Input: part model. Units: mm. Frame: model coordinates. A direction names the side the tool comes from. Coordinates: 2 decimals unless noted, no trailing zeros. Write each loop counter-clockwise with the first axis right and the second up, starting at its lowest first coordinate (ties: lowest second). Pieces come first, ordered by that corner, then holes. Notation, with made-up numbers: (19, -21) -> (42, -21) arc R16 ccw to (42, -13) -> close; hole circle Ø1 at (-6.5, -28.75). An arc over 180 degrees is marked (long way). Use one line per item in the form item = value. Start each with the question number.
(1) Cut plane B-B on y = 20.5. Return the cut outline in (x, z).
(2) Ray query, line 1 along X through (y, z) = (-43, 30); line 2 along X through (y, z) = (-16.5, 34.5); line 3 along X through (y, z) = (-49.5, 23.5). Return the intervals inside material, ascending.
(3) Cut plane A-A on x = -52.5. Return the cut outline in (y, z), plus the area to 3 significant figures.
(4) Cut plane D-D on y = 48.5. Return the cut outline in (x, z), plus the area to 3 significant figures.
(5) Set-up query: faces 5 (the face through (29.11, 26.443, 19.72)), 6 (the face through (63.35, -12.65, 20.28)). Return all of +Z, -Z, +X, -X, +Y, -Y with unobstructed straight access to the full face (end or side cutting, diameter ignored); none if empty.
(6) First-contact query: pin 1 (10 mm diameter, centred on x = -55, y = 3.5, fed in from +Z); pin 2 (3 mm diameter, centred on x = -56, z = 8.5, fed in from +Y); pin 3 (3 mm diameter, centred on x = 38.5, z = 4.5, fed in from -Y); pin 4 (4 mm diameter, centred on x = -22.5, z = 7, fed in from +Y). Flat tips, straight axial feed; report the tip coordinate or a pass-through.
(7) Pull-direction query (X, two-part tool) for faces 1 (the face through (-41.248, -11.06, 20.28)), 2 (the face through (-37.988, 18.432, 19.72)), 3 (the face through (-8.77, -99.04, 19.72)), 4 (the face through (-18, -41, 40)); classes: released by +X, released by -X, zero draft, split by the parting line, or undercut.
(8) Cut plane C-C on z = 25. Return the cut outline in (x, y), plus the area to 3 significant figures.
```python
from build123d import *

# Parameters (mm, degrees)
BOSS_EXTRUDE1_DEPTH = 40
SKETCH2_R           = 22.631847918
SKETCH2_R_2         = 28.776537022
CUT_EXTRUDE2_DEPTH  = 40


with BuildPart() as part:
    # Sketch1 → Boss-Extrude1 (new body)
    with BuildSketch(Plane.XY):
        Polygon((-147.819271396, 6.108234355), (-74.927674757, 40.314346744), (0, -4.072156237), (59.046265434, 57.824618563), (108.319355899, -8.551528097), (47.237012347, -105.061630909), (-66.37614666, -92.845162199), align=None)
    extrude(amount=BOSS_EXTRUDE1_DEPTH)

    # Sketch2 → Cut-Extrude2 (cut)
    with BuildSketch(Plane.XY.offset(40)):
        with Locations((51.179511342, -31.732249283)):
            Circle(SKETCH2_R)
        with Locations((-68.695439343, -19.703274992)):
            Circle(SKETCH2_R_2)
    extrude(amount=-CUT_EXTRUDE2_DEPTH, mode=Mode.SUBTRACT)


solid = part.part
```
Values:
q1.outline = (-117.15, 0) -> (-41.48, 0) -> (-41.48, 40) -> (-117.15, 40) -> close; (23.44, 0) -> (86.75, 0) -> (86.75, 40) -> (23.44, 40) -> close
q2.line_1 = -107.4 to -85.59, -51.8 to 31.55, 70.81 to 86.52
q2.line_2 = -129.21 to -97.29, -40.1 to 34.44, 67.92 to 103.29
q2.line_3 = -102.05 to 37.16, 65.2 to 82.4
q3.outline = (-94.34, 0) -> (-43.49, 0) -> (-43.49, 40) -> (-94.34, 40) -> close; (4.08, 0) -> (27.03, 0) -> (27.03, 40) -> (4.08, 40) -> close
q3.area = 2,950 mm2
q4.outline = (50.15, 0) -> (65.97, 0) -> (65.97, 40) -> (50.15, 40) -> close
q4.area = 633 mm2
q5.face_5 = +Z, -Z, +Y
q5.face_6 = +Z, -Z
q6.pin_1 = 40
q6.pin_2 = 29.99
q6.pin_3 = -104.28
q6.pin_4 = 10.44
q7.face_1 = undercut
q7.face_2 = undercut
q7.face_3 = released by -X
q7.face_4 = zero draft
q8.outline = (-147.82, 6.11) -> (-66.38, -92.85) -> (47.24, -105.06) -> (108.32, -8.55) -> (59.05, 57.82) -> (0, -4.07) -> (-74.93, 40.31) -> close; hole circle Ø57.55 at (-68.7, -19.7); hole circle Ø45.26 at (51.18, -31.73)
q8.area = 19,900 mm2
